```python
from build123d import *

# Parameters (mm, degrees)
SKETCH1_W           = 56.388
SKETCH1_H           = 56.388
BOSS_EXTRUDE1_DEPTH = 54.356
CUT_EXTRUDE1_DEPTH  = 49.276
FILLET2_R           = 5.08
FILLET3_R           = 2.54
SKETCH6_R           = 19.05
BOSS_EXTRUDE2_DEPTH = 1.524
BOSS_EXTRUDE3_DEPTH = 18.542
SKETCH10_R          = 2.413
CUT_EXTRUDE2_DEPTH  = 18.542
CHAMFER1_SIZE       = 0.508
CHAMFER2_SIZE       = 0.508
CHAMFER3_SIZE       = 2.54


with BuildPart() as part:
    # Sketch1 → Boss-Extrude1 (new body)
    with BuildSketch(Plane.XY):
        with Locations((28.194, -28.194)):
            Rectangle(SKETCH1_W, SKETCH1_H)
    extrude(amount=BOSS_EXTRUDE1_DEPTH)

    # Sketch3 → Cut-Extrude1 (cut)
    with BuildSketch(Plane.XY.offset(54.356)):
        Polygon((0, 0), (10.922, 0), (7.62, -7.62), (0, -10.922), align=None)
        Polygon((56.388, 0), (56.388, -10.922), (48.768, -7.62), (45.466, 0), align=None)
        Polygon((0, -56.388), (10.922, -56.388), (7.62, -48.768), (0, -45.466), align=None)
        Polygon((56.388, -56.388), (56.388, -45.466), (48.768, -48.768), (45.466, -56.388), align=None)
    extrude(amount=-CUT_EXTRUDE1_DEPTH, mode=Mode.SUBTRACT)

    # Fillet2
    fillet2_edges = [part.edges().sort_by_distance(p)[0] for p in [
        (0, 0, 2.54),
        (7.62, -7.62, 29.718),
        (56.388, 0, 2.54),
        (48.768, -7.62, 29.718),
        (0, -56.388, 2.54),
        (7.62, -48.768, 29.718),
        (56.388, -56.388, 2.54),
        (48.768, -48.768, 29.718),
    ]]
    fillet(fillet2_edges, radius=FILLET2_R)

    # Fillet3
    fillet3_edges = [part.edges().sort_by_distance(p)[0] for p in [
        (0, -10.922, 29.718),
        (10.922, 0, 29.718),
        (45.466, 0, 29.718),
        (56.388, -10.922, 29.718),
        (0, -45.466, 29.718),
        (10.922, -56.388, 29.718),
        (45.466, -56.388, 29.718),
        (56.388, -45.466, 29.718),
    ]]
    fillet(fillet3_edges, radius=FILLET3_R)

    # Sketch6 → Boss-Extrude2 (add)
    with BuildSketch(Plane(origin=(0, 0, 0), x_dir=(-1, 0, 0), z_dir=(0, 0, -1))):
        with Locations(Location((-28.194, -28.194, 0), (0, 0, 180))):
            Circle(SKETCH6_R)
    extrude(amount=BOSS_EXTRUDE2_DEPTH)

    # Sketch8 → Boss-Extrude3 (add)
    with BuildSketch(Plane(origin=(0, 0, -1.524), x_dir=(-1, 0, 0), z_dir=(0, 0, -1))):
        with BuildLine():
            Line((-30.861, -26.471288184), (-30.861, -29.916711816))
            ThreePointArc((-30.861, -29.916711816), (-25.019, -28.194), (-30.861, -26.471288184))
        make_face()
    extrude(amount=BOSS_EXTRUDE3_DEPTH)

    # Sketch10 → Cut-Extrude2 (cut)
    with BuildSketch(Plane(origin=(0, 0, 0), x_dir=(-1, 0, 0), z_dir=(0, 0, -1))):
        with Locations((-51.562, -4.826)):
            Circle(SKETCH10_R)
        with Locations((-4.826, -4.826)):
            Circle(SKETCH10_R)
        with Locations((-51.562, -51.562)):
            Circle(SKETCH10_R)
        with Locations((-4.826, -51.562)):
            Circle(SKETCH10_R)
    extrude(amount=-CUT_EXTRUDE2_DEPTH, mode=Mode.SUBTRACT)

    # Chamfer1
    chamfer1_edges = [part.edges().sort_by_distance(p)[0] for p in [
        (53.975, -4.826, 0),
        (7.239, -4.826, 0),
        (53.975, -51.562, 0),
        (7.239, -51.562, 0),
    ]]
    chamfer(chamfer1_edges, length=CHAMFER1_SIZE)

    # Chamfer2
    chamfer2_edges = [part.edges().sort_by_distance(p)[0] for p in [
        (25.019, -28.194, -20.066),
    ]]
    chamfer(chamfer2_edges, length=CHAMFER2_SIZE - 0.0001)  # a hair under: the kernel refuses the full size

    # Chamfer3
    chamfer3_edges = [part.edges().sort_by_distance(p)[0] for p in [
        (47.049244866, -3.653641998, 54.356),
        (52.734358002, -47.049244866, 54.356),
        (56.388, -28.194, 54.356),
        (28.194, 0, 54.356),
        (3.653641998, -9.338755134, 54.356),
        (0, -28.194, 54.356),
        (9.338755134, -52.734358002, 54.356),
        (28.194, -56.388, 54.356),
        (0.416700193, -11.19557153, 54.356),
        (11.19557153, -0.416700193, 54.356),
        (0.416700193, -45.19242847, 54.356),
        (11.19557153, -55.971299807, 54.356),
        (45.19242847, -55.971299807, 54.356),
        (55.971299807, -45.19242847, 54.356),
        (55.971299807, -11.19557153, 54.356),
        (45.19242847, -0.416700193, 54.356),
        (3.653641998, -47.049244866, 54.356),
        (47.049244866, -52.734358002, 54.356),
        (52.734358002, -9.338755134, 54.356),
        (9.338755134, -3.653641998, 54.356),
        (7.349463554, -49.038536446, 54.356),
        (49.038536446, -49.038536446, 54.356),
        (49.038536446, -7.349463554, 54.356),
        (7.349463554, -7.349463554, 54.356),
    ]]
    chamfer(chamfer3_edges, length=CHAMFER3_SIZE)


solid = part.part
```
Model file for the job. Use its own axes, mm. A direction names the side the tool comes from. Coordinates: 2 decimals unless noted, no trailing zeros. Loops run counter-clockwise (first coordinate to the right, second up) from the corner with the lowest first, then second, coordinate; pieces in that order, holes last. Notation, with made-up numbers: (-32.5, 85) - (18.5, 85) arc R32 ccw to (18.5, 119) - close; hole circle Ø5 at (78.25, 72). An arc over 180 degrees is marked (long way). Write item = value, one per line. Start each with the question number.
Item 1: Pull direction X, two halves, no side cores. Call faces 4 (the face through (25.02, -28.31, -10.41)), 5 (the face through (7.3, -7.4, 28.1)), 6 (the face through (5.349, -53.918, 2.762)): +X half, -X half, draft (parallel to the pull), parting line (faces both ways), or undercut.
Item 2: Drop flat-ended pins along their axis: pin 1 Ø4 at (x, z) = (49, 10) entering from -Y; pin 2 Ø7.5 at (x, y) = (4.826, -51.562) entering from +Z; pin 3 Ø17 at (x, y) = (37.5, -36.5) entering from -Z. Give the stop position or say it passes through.
Item 3: Saw through at D-D, the plane z = -6.5. List the corners of the cut face in (x, y) (3 decimals).
Item 4: Saw through at C-C, the plane x = 15.5. List the corners of the cut face in (y, z), then the cut area to 3 significant figures.
Item 5: Saw through at B-B, the plane y = -16.5. List the corners of the cut face in (x, z).
Item 6: Saw through at A-A, the plane z = 19.5. List the corners of the cut face in (x, y), then the cut area to 3 significant figures.
Item 7: Wall check: probe 1 along Z at (x, y) = (37, -13.5); probe 2 along X at (y, z) = (-52, 3); probe 3 along Z at (x, y) = (26.5, -50.5). Give the ranges that are in metal, low to high. Write a range as [from, to].
Item 8: 3-axis set-ups, long thin cutter, end or side, ignore diameter. For faces 1 (the face through (47.06, -3.68, 28.78)), 2 (the face through (22, -9, 0)), 3 (the face through (5, -2, 5.08)): which of +Z, -Z, +X, -X, +Y, -Y reach the whole face in a straight line?
Answers:
q1.face_4 = parting line
q1.face_5 = -X half
q1.face_6 = undercut
q2.pin_1 = -52.85
q2.pin_2 = 52
q2.pin_3 = -1.52
q3.outline = (30.861, -29.917) - (30.861, -26.471) arc R3.175 ccw (long way) to start
q4.outline = (-56.39, 0) - (-42.4, 0) - (-42.4, -1.52) - (-13.99, -1.52) - (-13.99, 0) - (0, 0) - (0, 51.82) - (-2.54, 54.36) - (-53.85, 54.36) - (-56.39, 51.82) - close
q4.area = 3,100 mm2
q5.outline = (0, 0) - (13.16, 0) - (13.16, -1.52) - (43.23, -1.52) - (43.23, 0) - (56.39, 0) - (56.39, 51.82) - (53.85, 54.36) - (2.54, 54.36) - (0, 51.82) - close
q6.outline = (0, -43.8) arc R2.54 ccw to (1.53, -46.13) - (5.78, -47.97) arc R5.08 cw to (8.42, -50.61) - (10.26, -54.86) arc R2.54 ccw to (12.59, -56.39) - (43.8, -56.39) arc R2.54 ccw to (46.13, -54.86) - (47.97, -50.61) arc R5.08 cw to (50.61, -47.97) - (54.86, -46.13) arc R2.54 ccw to (56.39, -43.8) - (56.39, -12.59) arc R2.54 ccw to (54.86, -10.26) - (50.61, -8.42) arc R5.08 cw to (47.97, -5.78) - (46.13, -1.53) arc R2.54 ccw to (43.8, 0) - (12.59, 0) arc R2.54 ccw to (10.26, -1.53) - (8.42, -5.78) arc R5.08 cw to (5.78, -8.42) - (1.53, -10.26) arc R2.54 ccw to (0, -12.59) - close
q6.area = 2,840 mm2
q7.probe_1 = [-1.52, 54.36]
q7.probe_2 = [0.05, 2.45], [7.2, 49.19], [53.93, 56.34]
q7.probe_3 = [0, 54.36]
q8.face_1 = +Z, +X, +Y
q8.face_2 = -Z
q8.face_3 = +Z, -X, +Y
